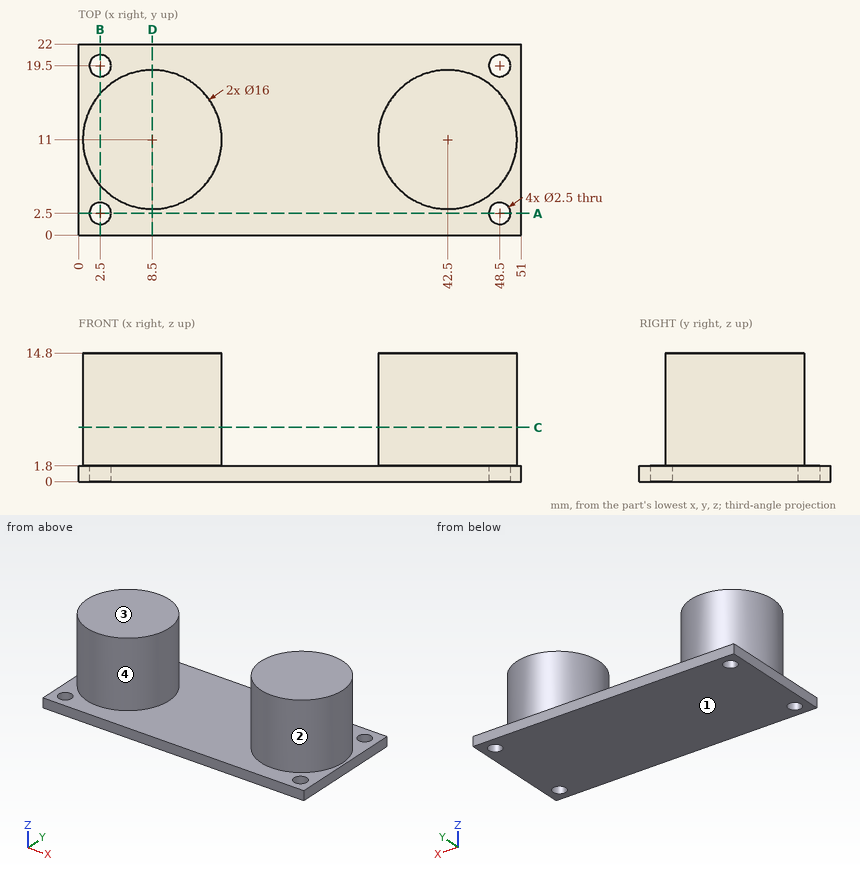
For this review, use the dimensioned drawing (mm, ordinates from the lowest corner) and the shaded views. A direction names the side the tool comes from. Coordinates: 2 decimals unless noted, no trailing zeros. Order: outer loops, then holes, each group sorted by start corner. A loop starts at its lowest first (then second) coordinate and runs counter-clockwise, first axis right, second up. Notation, with made-up numbers: (71.5, 67) - (129.5, 67) arc R25 cw to (129.5, 82) - close; hole circle Ø6 at (-6, -30.75). An arc over 180 degrees is marked (long way). Use one line per item in the form item = value.
Q1. For P1, Ø4, axis at x = 37.5, y = 10, coming from the -Z side; P2, Ø6, axis at y = 12, z = 9, coming from the -X side; P3, Ø3, axis at x = 48.5, y = 2.5, coming from the +Z side, all flat-tipped, find the tip position at first contact; note any pin that passes through.
Checked values:
P1 = 0
P2 = 0.5
P3 = 1.8
Q2. For probe 1 along Y at (x, z) = (48.5, 0.9); probe 2 along X at (y, z) = (10.75, 5.5); probe 3 along X at (y, z) = (6.75, 6), list the stretches that pass through material, from the lowest coordinate up. Write a range as from..to.
Checked values:
probe_1 = 0..1.25, 3.75..18.25, 20.75..22
probe_2 = 0.5..16.5, 34.5..50.5
probe_3 = 1.72..15.28, 35.72..49.28
Q3. Consider section C-C (z = 6.25). Give the boundary of the cut face in (x, y), then the cut area to 3 significant figures.
Checked values:
outline = circle Ø16 at (8.5, 11); circle Ø16 at (42.5, 11)
area = 402 mm2
Q4. Consider section B-B (x = 2.5). Give the boundary of the cut face in (y, z).
Checked values:
outline = (0, 0) - (1.25, 0) - (1.25, 1.8) - (0, 1.8) - close; (3.75, 0) - (18.25, 0) - (18.25, 1.8) - (16.29, 1.8) - (16.29, 14.8) - (5.71, 14.8) - (5.71, 1.8) - (3.75, 1.8) - close; (20.75, 0) - (22, 0) - (22, 1.8) - (20.75, 1.8) - close
Q5. For the marked faces 3 and 4, list the 3-axis set-ups (+Z, -Z, +X, -X, +Y, -Y) from which the entire face can be reached by the end or side of a thin tool; tool diameter is ignored.
Checked values:
face_3 = +Z, +X, -X, +Y, -Y
face_4 = +Z
Q6. Consider section A-A (y = 2.5). Give the boundary of the cut face in (x, z), then the cut area to 3 significant figures.
Checked values:
outline = (0, 0) - (1.25, 0) - (1.25, 1.8) - (0, 1.8) - close; (3.75, 0) - (47.25, 0) - (47.25, 1.8) - (3.75, 1.8) - close; (49.75, 0) - (51, 0) - (51, 1.8) - (49.75, 1.8) - close
area = 82.8 mm2
Q7. Consider section D-D (x = 8.5). Give the boundary of the cut face in (y, z), then the cut area to 3 significant figures.
Checked values:
outline = (0, 0) - (22, 0) - (22, 1.8) - (19, 1.8) - (19, 14.8) - (3, 14.8) - (3, 1.8) - (0, 1.8) - close
area = 248 mm2
Q8. Draft analysis for pull direction X (two halves, no side actions). For the marked faces 1 and 2, state which applies: +X half, -X half, draft (parallel to the pull), parting line (faces both ways), or undercut.
Checked values:
face_1 = draft
face_2 = undercut
